Can you work these out from the model? Positions are in its coordinate system, mm. A direction names the side the tool comes from. Coordinates: 2 decimals unless noted, no trailing zeros. Loops run counter-clockwise (first coordinate to the right, second up) from the corner with the lowest first, then second, coordinate; pieces in that order, holes last.
```python
from build123d import *

# Parameters (mm, degrees)
SKETCH1_W           = 35
SKETCH1_H           = 25
BOSS_EXTRUDE1_DEPTH = 5
SKETCH2_W           = 5
SKETCH2_H           = 25
BOSS_EXTRUDE2_DEPTH = 40
SKETCH3_R           = 6
CUT_EXTRUDE1_DEPTH  = 59.736700622
SKETCH4_R           = 2
CUT_EXTRUDE2_DEPTH  = 60.581876439


with BuildPart() as part:
    # Sketch1 → Boss-Extrude1 (new body)
    with BuildSketch(Plane.XY):
        with Locations((17.5, 12.5)):
            Rectangle(SKETCH1_W, SKETCH1_H)
    extrude(amount=BOSS_EXTRUDE1_DEPTH)

    # Sketch2 → Boss-Extrude2 (add)
    with BuildSketch(Plane.XY.offset(5)):
        with Locations((32.5, 12.5)):
            Rectangle(SKETCH2_W, SKETCH2_H)
    extrude(amount=BOSS_EXTRUDE2_DEPTH)

    # Sketch3 → Cut-Extrude1 (cut, through all)
    with BuildSketch(Plane.XY.offset(5)):
        with Locations((12.5, 12.5)):
            Circle(SKETCH3_R)
    extrude(amount=-CUT_EXTRUDE1_DEPTH, mode=Mode.SUBTRACT)

    # Sketch4 → Cut-Extrude2 (cut, through all)
    with BuildSketch(Plane.ZY.offset(-30)):
        with Locations(Location((15, 12.5, 0), (0, 0, 270))):
            Circle(SKETCH4_R)
        with Locations(Location((35, 12.5, 0), (0, 0, 270))):
            Circle(SKETCH4_R)
    extrude(amount=-CUT_EXTRUDE2_DEPTH, mode=Mode.SUBTRACT)


solid = part.part
```
Item 1: I'm going to push flat-ended pins straight in: P1, Ø4.5, axis at y = 12.5, z = 15, coming from the +X side; P2, Ø12.5, axis at y = 18, z = 34, coming from the -X side. Where does each tip first touch, or does it pass through?
Results are:
P1: stops at x = 35
P2: stops at x = 30
Item 2: Suppose I cut it at A-A, the plane x = 12.5. Please give me the cut outline in (y, z), plus the area to 3 significant figures.
Results are:
outline: (0, 0) - (6.5, 0) - (6.5, 5) - (0, 5) - close; (18.5, 0) - (25, 0) - (25, 5) - (18.5, 5) - close
area: 65.0 mm2
Item 3: Suppose I cut it at C-C, the plane z = 15. Please give me the cut outline in (x, y).
Results are:
outline: (30, 0) - (35, 0) - (35, 10.5) - (30, 10.5) - close; (30, 14.5) - (35, 14.5) - (35, 25) - (30, 25) - close
Item 4: On a 3-axis mill with a long thin cutter (end or side, diameter ignored), from which of +Z, -Z, +X, -X, +Y, -Y can I reach the whole of each face in a straight line? I mean faces 1 (the face through (0, 12, 2)), 2 (the face through (18.1, 15.5, 5)). Say none if no direction works.
Results are:
face 1: +Z, -Z, -X, +Y, -Y
face 2: +Z, -X, +Y, -Y
Item 5: Suppose I cut it at D-D, the plane y = 17.5. Please give me the cut outline in (x, z).
Results are:
outline: (0, 0) - (9.18, 0) - (9.18, 5) - (0, 5) - close; (15.82, 0) - (35, 0) - (35, 45) - (30, 45) - (30, 5) - (15.82, 5) - close
Item 6: I need wall thicknesses on line 1 along Z through (x, y) = (33.45, 12.5); line 2 along Y through (x, z) = (12.5, 1.1); line 3 along X through (y, z) = (18.5, 35). Which ranges of each line are inside material? Lowest first, please.
Results are:
line 1: z = 0 to 13, 17 to 33, 37 to 45
line 2: y = 0 to 6.5, 18.5 to 25
line 3: x = 30 to 35
Item 7: We'd pull the mould along Y, two halves only. Please class faces 3 (the face through (30.4, 0, 14.1)), 4 (the face through (30, 12, 25)), 5 (the face through (15.269, 7.177, 2.535)): +Y half, -Y half, draft (parallel to the pull), parting line (faces both ways), or undercut.
Results are:
face 3: -Y half
face 4: draft
face 5: undercut
Item 8: Suppose I cut it at B-B, the plane y = 12.5. Please give me the cut outline in (x, z).
Results are:
outline: (0, 0) - (6.5, 0) - (6.5, 5) - (0, 5) - close; (18.5, 0) - (35, 0) - (35, 13) - (30, 13) - (30, 5) - (18.5, 5) - close; (30, 17) - (35, 17) - (35, 33) - (30, 33) - close; (30, 37) - (35, 37) - (35, 45) - (30, 45) - close
